For this review, use the dimensioned drawing (mm, ordinates from the lowest corner) and the shaded views. A direction names the side the tool comes from. Coordinates: 2 decimals unless noted, no trailing zeros. Write each loop counter-clockwise with the first axis right and the second up, starting at its lowest first coordinate (ties: lowest second). Pieces come first, ordered by that corner, then holes. Notation, with made-up numbers: (7, 27) -> (29, 27) arc R7 cw to (29, 39) -> close; hole circle Ø6 at (61.25, 33.5). An arc over 180 degrees is marked (long way). Put each result on its own line as item: value. Start each with the question number.
Item 1: Consider section A-A on x = 5.5. Give the boundary of the cut face in (y, z), and give its area (3 significant figures).
Item 2: Consider section C-C on z = 23. Give the boundary of the cut face in (x, y).
Item 3: Consider section B-B on y = 28. Give the boundary of the cut face in (x, z).
Item 4: Insertion check: P1, Ø12.5, axis at y = 11, z = 17.5, coming from the +X side; P2, Ø10, axis at x = 57.5, y = 24, coming from the -Z side. Each pin has a flat end and moves straight along its axis. Give the tip position at first contact, or say it passes through.
Item 5: For the marked faces 1 and 2, list the 3-axis set-ups (+Z, -Z, +X, -X, +Y, -Y) from which the entire face can be reached by the end or side of a thin tool; tool diameter is ignored.
Item 6: Consider section D-D on y = 20. Give the boundary of the cut face in (x, z).
Item 7: To check wall thickness, follow L1, parallel to Y at x = 43, z = 28.2; L2, parallel to X at y = 30, z = 13; L3, parallel to X at y = 15.5, z = 25.5. State the ranges of each line that lie inside material, in increasing order.
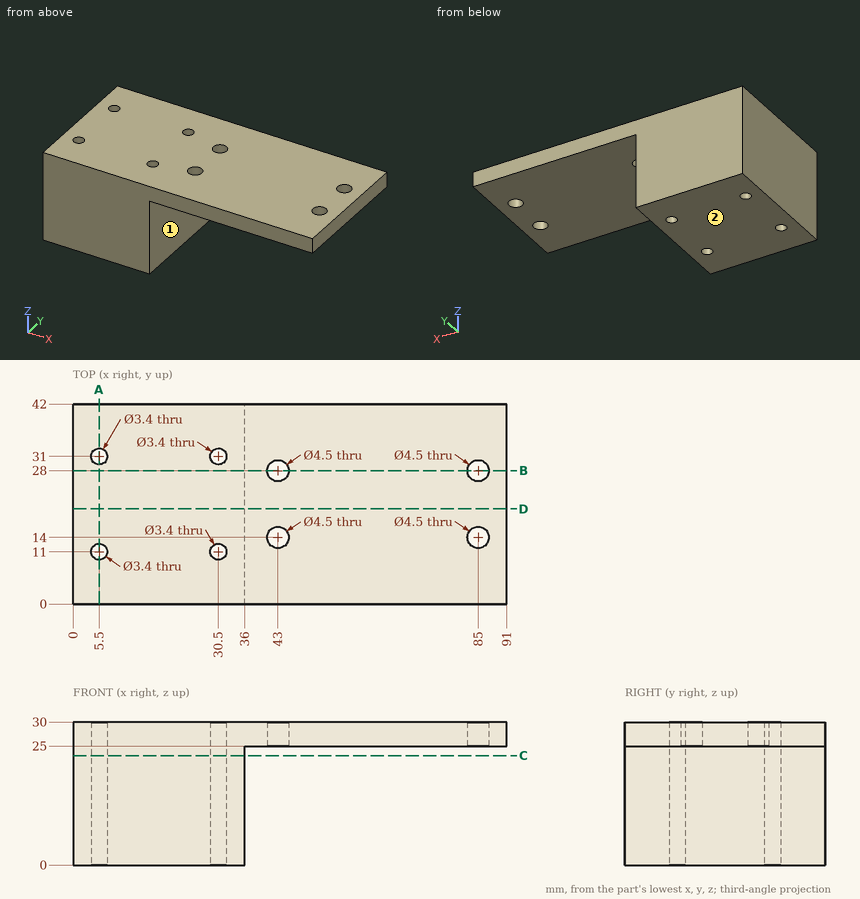
Return value:
1. outline: (0, 0) -> (9.3, 0) -> (9.3, 30) -> (0, 30) -> close; (12.7, 0) -> (29.3, 0) -> (29.3, 30) -> (12.7, 30) -> close; (32.7, 0) -> (42, 0) -> (42, 30) -> (32.7, 30) -> close
1. area: 1,060 mm^2
2. outline: (0, 0) -> (36, 0) -> (36, 42) -> (0, 42) -> close; hole circle Ø3.4 at (5.5, 11); hole circle Ø3.4 at (5.5, 31); hole circle Ø3.4 at (30.5, 11); hole circle Ø3.4 at (30.5, 31)
3. outline: (0, 0) -> (36, 0) -> (36, 25) -> (40.75, 25) -> (40.75, 30) -> (0, 30) -> close; (45.25, 25) -> (82.75, 25) -> (82.75, 30) -> (45.25, 30) -> close; (87.25, 25) -> (91, 25) -> (91, 30) -> (87.25, 30) -> close
4. P1: x = 36
4. P2: z = 25
5. face 1: -Z, +X, +Y, -Y
5. face 2: -Z, +X, -X, +Y, -Y
6. outline: (0, 0) -> (36, 0) -> (36, 25) -> (91, 25) -> (91, 30) -> (0, 30) -> close
7. L1: 0 to 11.75, 16.25 to 25.75, 30.25 to 42
7. L2: 0 to 4.13, 6.87 to 29.13, 31.87 to 36
7. L3: 0 to 41.32, 44.68 to 83.32, 86.68 to 91
